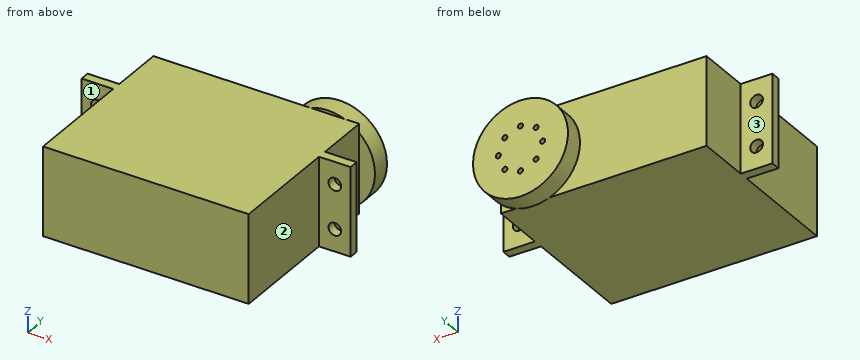
Autodesk Inventor part; units mm, degrees
ref_plane "YZ Plane" through (0, 0, 0) normal (1, 0, 0) x (0, 1, 0)
ref_plane "XZ Plane" through (0, 0, 0) normal (0, 1, 0) x (-1, 0, 0)
ref_plane "XY Plane" through (0, 0, 0) normal (0, 0, 1) x (1, 0, 0)
sketch "Sketch1" plane through (0, 0, 0) normal (0, 1, 0) x (-1, 0, 0)
  line L0 (32.5, 14) -> (19.5, 14)
  line L1 (-32.5, 14) -> (-32.5, -14)
  line L2 (-32.5, -14) -> (19.5, -14)
  line L3 (32.5, -14) -> (32.5, 14)
  line L4 (32.5, 14) -> (-32.5, -14) construction
  line L5 (-32.5, 14) -> (32.5, -14) construction
  line L6 (19.5, 14) -> (-32.5, 14)
  line L7 (19.5, -14) -> (32.5, -14)
  point P0 (0, 0)
  point P1 (32.5, 7.3274)
  point P2 (32.5, -11.3274)
  dimension "d0" = 65
  dimension "d1" = 28
extrude "Extrusion1" add sketch "Sketch1" along normal blind 55
sketch "Sketch2" plane through (0, 55, 0) normal (0, 1, 0) x (1, 0, 0)
  circle A0 centre (22.5, 0) radius 15
  line L0 (32.5, -14) -> (32.5, 14)
  line L1 (-32.5, -14) -> (32.5, -14)
  point P0 (0, 0)
  point P1 (-8.5, -16)
  dimension "d4" = 10
  dimension "d5" = 30
  dimension "d28" = 14
extrude "Extrusion2" add sketch "Sketch2" along normal blind 6 contours A0 L0 | L0 A0 L1 | L1 A0 picked at (24.6253, 2.0919)
sketch "Sketch3" plane through (22.5, 61, 0) normal (0, 1, 0) x (1, 0, 0)
  circle A0 centre (-7, 0) radius 0.8
  circle A1 centre (0, 0) radius 15
  circle A2 centre (-4.9497, -4.9497) radius 0.8
  circle A3 centre (0, -7) radius 0.8
  circle A4 centre (4.9497, -4.9497) radius 0.8
  circle A5 centre (7, 0) radius 0.8
  circle A6 centre (4.9497, 4.9497) radius 0.8
  circle A7 centre (0, 7) radius 0.8
  circle A8 centre (-4.9497, 4.9497) radius 0.8
  point P0 (-22.5, 0)
  dimension "d12" = 1.6
  dimension "d14" = 7
  dimension "d17" = 360
extrude "Extrusion3" cut sketch "Sketch3" against normal up to surface (6 mm away) contours A0 | A2 | A3 | A4 | A5 | A6 | A7 | A8
sketch "Sketch4" plane through (0, 55, 0) normal (0, 1, 0) x (1, 0, 0)
  circle A0 centre (-37.5, -7) radius 2
  circle A1 centre (37.5, -7) radius 2
  circle A2 centre (37.5, 7) radius 2
  circle A3 centre (-37.5, 7) radius 2
  line L0 (-32.5, -14) -> (32.5, -14)
  line L1 (32.5, -14) -> (32.5, 14)
  line L2 (-32.5, 14) -> (-32.5, -14)
  line L3 (-32.5, 14) -> (-42.5, 14)
  line L4 (-42.5, 14) -> (-42.5, -14)
  line L5 (-42.5, -14) -> (-32.5, -14)
  line L6 (-32.5, -14) -> (-32.5, 14)
  line L7 (32.5, 14) -> (42.5, 14)
  line L8 (42.5, 14) -> (42.5, -14)
  line L9 (42.5, -14) -> (32.5, -14)
  line L10 (32.5, -14) -> (32.5, 14)
  point P0 (0, 0)
  point P1 (-8.5, -16)
  point P2 (29.5, -14)
  point P3 (32.5, -11)
  point P4 (32.5, 11)
  dimension "d21" = 4
  dimension "d22" = 14
  dimension "d23" = 7
  dimension "d29" = 5
  dimension "d30" = 5
  dimension "d31" = 5
  dimension "d32" = 5
extrude "Extrusion4" add sketch "Sketch4" against normal blind 20
sketch "Sketch5" plane through (0, 55, 0) normal (0, 1, 0) x (1, 0, 0)
  line L0 (42.5, 14) -> (-42.5, 14)
  line L1 (-32.5, 14) -> (-32.5, -14)
  line L2 (-42.5, 14) -> (-32.5, 14)
  line L3 (-32.5, 14) -> (-32.5, -14)
  line L4 (-32.5, -14) -> (-42.5, -14)
  line L5 (-42.5, -14) -> (-42.5, 14)
  line L6 (32.5, -14) -> (32.5, 14)
  line L7 (42.5, 14) -> (42.5, -14)
  line L8 (32.5, -14) -> (42.5, -14)
  line L9 (42.5, -14) -> (42.5, 14)
  line L10 (42.5, 14) -> (32.5, 14)
  line L11 (32.5, 14) -> (32.5, -14)
  point P0 (0, 0)
extrude "Extrusion5" cut sketch "Sketch5" against normal blind 17
equation "\"d30\" = d29"
equation "\"d31\" = d30"
equation "\"d32\" = d29"
properties part number "servo" material "Aluminum"
Model file for the job. Use its own axes, mm. Face numbers are marked on the shaded views. A direction names the side the tool comes from. Coordinates: 2 decimals unless noted, no trailing zeros. Write each loop counter-clockwise with the first axis right and the second up, starting at its lowest first coordinate (ties: lowest second). Pieces come first, ordered by that corner, then holes. Notation, with made-up numbers: (22, 79.5) -> (55, 79.5) arc R30 ccw to (55, 105.5) -> close; hole circle Ø7 at (52, 14). An arc over 180 degrees is marked (long way). One line per item, written item: value. Start each with the question number.
1) Slice it at B-B on y = 11. Write the cut outline in (x, z), then the cut area to 3 significant figures.
2) Flat gauge pins, fed straight in: pin 1 Ø0.5 at (x, z) = (29, -0.5) entering from +Y; pin 2 Ø11 at (x, z) = (-38.5, 5) entering from -Y; pin 3 Ø4 at (x, y) = (-18.5, 49) entering from -Z; pin 4 Ø6 at (x, z) = (-17.5, 8) entering from +Y. Where does each tip first touch, or does it go through?
3) Slice it at A-A on z = 12.75. Write the cut outline in (x, y).
4) Slice it at C-C on x = -9.5. Write the cut outline in (y, z).
5) Which spindle directions (+Z, -Z, +X, -X, +Y, -Y) get a long thin tool onto all of the face, cutting with end or side? Do the marked faces 1, 2 and 3. Say none if no direction does.
6) Probe probe 1 along X at (y, z) = (36.5, -7); probe 2 along Z at (x, y) = (-37.5, 36.1); probe 3 along Z at (x, y) = (37, 36). List the from-to ranges inside material, lowest first.
Answers follow:
1. outline: (-32.5, -14) -> (32.5, -14) -> (32.5, 14) -> (-32.5, 14) -> close
1. area: 1,820 mm2
2. pin 1: y = 61
2. pin 2: y = 35
2. pin 3: z = -14
2. pin 4: y = 55
3. outline: (-42.5, 35) -> (-32.5, 35) -> (-32.5, 0) -> (32.5, 0) -> (32.5, 35) -> (42.5, 35) -> (42.5, 38) -> (32.5, 38) -> (32.5, 55) -> (30.4, 55) -> (30.4, 61) -> (14.6, 61) -> (14.6, 55) -> (-32.5, 55) -> (-32.5, 38) -> (-42.5, 38) -> close
4. outline: (0, -14) -> (55, -14) -> (55, 14) -> (0, 14) -> close
5. face 1: +Z, -Z, -X, -Y
5. face 2: +Z, -Z, +X, -Y
5. face 3: +Z, -Z, -X, +Y
6. probe 1: -42.5 to -39.5, -35.5 to 35.5, 39.5 to 42.5
6. probe 2: -14 to -9, -5 to 5, 9 to 14
6. probe 3: -14 to -8.94, -5.06 to 5.06, 8.94 to 14
